Could you check a few things on this drawing? It's one solid part, dimensions in mm from its lowest x, y, z. Round coordinates to 2 decimals unless told otherwise and drop trailing zeros. Write each loop counter-clockwise with the first axis right and the second up, starting at its lowest first coordinate (ties: lowest second). Pieces come first, ordered by that corner, then holes. Notation, with made-up numbers: (33.5, -28) - (39.5, -28) arc R22 ccw to (39.5, 3) - close; hole circle Ø1 at (14, -20.5). An arc over 180 degrees is marked (long way). Put each result on its own line as item: value.
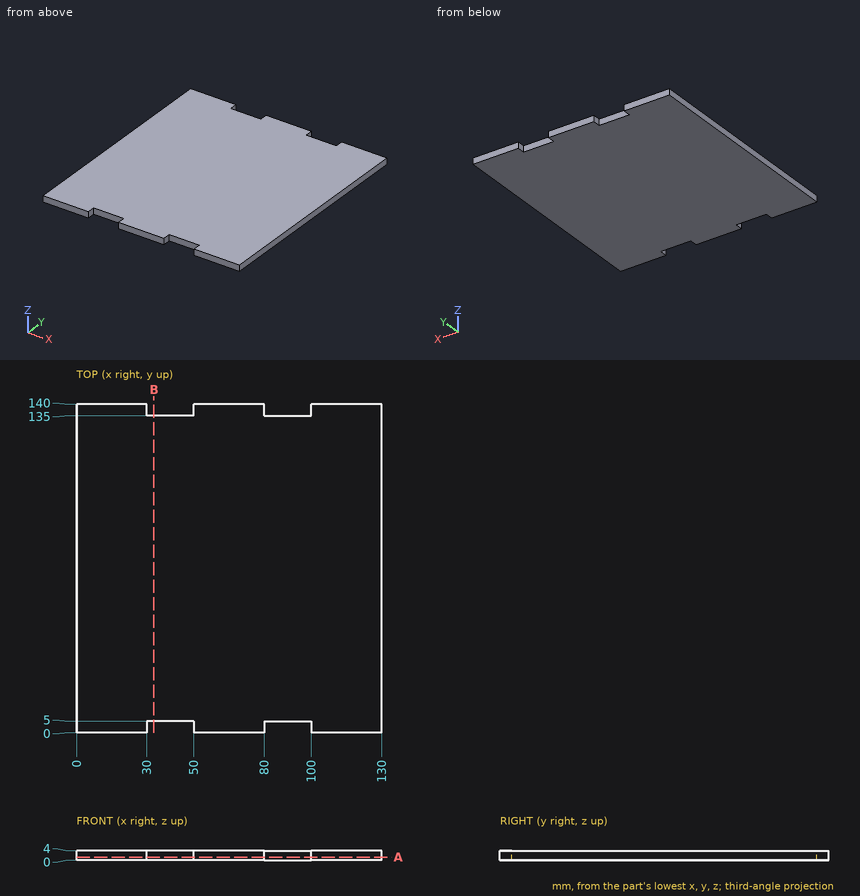
(1) I'm going to push a flat-ended pin straight in: pin 1 (1.2 mm diameter, centred on x = 94, z = 2, fed in from -Y). Where does the tip first touch, or does it pass through?
Values found:
pin 1: stops at y = 5
(2) Imagine slicing it at B-B, the plane x = 33. List the corners of the cut face in (y, z) for me.
Values found:
outline: (5, 0) - (135, 0) - (135, 4) - (5, 4) - close
(3) Please list where this line runs through material, in increasing order: probe 1 along Y at (x, z) = (90.5, 2.5). Write a range as from..to.
Values found:
probe 1: y = 5..135
(4) Imagine slicing it at A-A, the plane z = 1.3. List the corners of the cut face in (x, y) for me, then the cut area to 3 significant figures.
Values found:
outline: (0, 0) - (30, 0) - (30, 5) - (50, 5) - (50, 0) - (80, 0) - (80, 5) - (100, 5) - (100, 0) - (130, 0) - (130, 140) - (100, 140) - (100, 135) - (80, 135) - (80, 140) - (50, 140) - (50, 135) - (30, 135) - (30, 140) - (0, 140) - close
area: 17,800 mm^2
